Could you check a few things on this model? Use its own coordinates, in mm. Face numbers are marked on the shaded views. A direction names the side the tool comes from. Coordinates: 2 decimals unless noted, no trailing zeros. Loops run counter-clockwise (first coordinate to the right, second up) from the corner with the lowest first, then second, coordinate; pieces in that order, holes last. Notation, with made-up numbers: M 86,40.25 L 141,40.25 A20 cw 141,73.25 Z; hole C 88,23 d6. An arc over 180 degrees is marked long. Write each question's results on one line, items separated by ' | '.
```python
from build123d import *

# Parameters (mm, degrees)
SKETCH1_R           = 10.16
BOSS_EXTRUDE1_DEPTH = 7.62
SKETCH2_R           = 1.5875
CUT_EXTRUDE4_DEPTH  = 17.263935563
CUT_EXTRUDE5_DEPTH  = 6.35


with BuildPart() as part:
    # Sketch1 → Boss-Extrude1 (new body)
    with BuildSketch(Plane(origin=(0, 0, 0), x_dir=(1, 0, 0), z_dir=(0, 1, 0))):
        with Locations(Location((0, 0, 0), (0, 0, 90))):
            Circle(SKETCH1_R)
    extrude(amount=BOSS_EXTRUDE1_DEPTH)

    # Sketch2 → Cut-Extrude4 (cut, through all)
    with BuildSketch(Plane(origin=(0, 7.62, 0), x_dir=(1, 0, 0), z_dir=(0, 1, 0))):
        with Locations(Location((0, 0, 0), (0, 0, 270))):
            Circle(SKETCH2_R)
    extrude(amount=-CUT_EXTRUDE4_DEPTH, mode=Mode.SUBTRACT)

    # Sketch5 → Cut-Extrude5 (cut)
    with BuildSketch(Plane(origin=(0, 7.62, 0), x_dir=(1, 0, 0), z_dir=(0, 1, 0))):
        Polygon((6.247359776, 1.137099745), (2.138922622, 5.978922145), (-4.108437154, 4.8418224), (-6.247359776, -1.137099745), (-2.138922622, -5.978922145), (4.108437154, -4.8418224), align=None)
    extrude(amount=-CUT_EXTRUDE5_DEPTH, mode=Mode.SUBTRACT)


solid = part.part
```
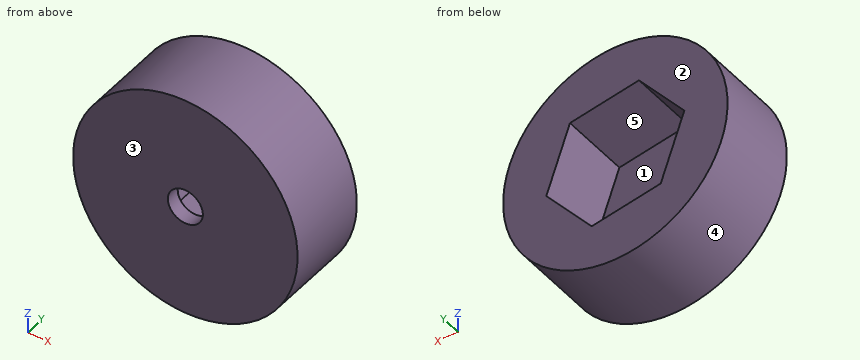
(1) Imagine slicing it at B-B, the plane y = 2.5. List the corners of the cut face in (x, z) for me, and give its area (3 significant figures).
Reported:
outline: C 0,0 d20.32; hole M -6.25,1.14 L -4.11,-4.84 L 2.14,-5.98 L 6.25,-1.14 L 4.11,4.84 L -2.14,5.98 Z | area: 220 mm2
(2) Imagine slicing it at C-C, the plane x = -5. List the corners of the cut face in (y, z) for me.
Reported:
outline: M 0,-8.84 L 7.62,-8.84 L 7.62,-2.35 L 1.27,-2.35 L 1.27,2.61 L 7.62,2.61 L 7.62,8.84 L 0,8.84 Z
(3) If we mould it in two halves opening along X, with no side actions, what happens to the marked faces 3, 4 and 5? For each: released by +X, released by -X, zero draft, split by the parting line, or undercut.
Reported:
face 3: zero draft | face 4: split by the parting line | face 5: undercut
(4) Please list where these lines run through material, in increasing order: probe 1 along X at (y, z) = (0.5, 0); probe 2 along X at (y, z) = (5.25, 0.25); probe 3 along Z at (x, y) = (1.25, 6.5). Write a range as from..to.
Reported:
probe 1: x = -10.16..-1.59, 1.59..10.16 | probe 2: x = -10.16..-5.93, 5.75..10.16 | probe 3: z = -10.08..-5.82, 5.36..10.08
(5) Will these pins go through, and if not, where does the flat tip stop? P1, Ø1.5, axis at y = 6.5, z = 2, coming from the +X side; P2, Ø1, axis at x = 3.5, y = 3, coming from the +Z side; P3, Ø3, axis at y = 6, z = 5.5, coming from the +X side; P4, Ø2.5, axis at x = 0, z = 0, coming from the -Y side.
Reported:
P1: stops at x = 10.08 | P2: stops at z = 9.71 | P3: stops at x = 9.34 | P4: passes through
(6) Which directions (+Z, -Z, +X, -X, +Y, -Y) give clear straight access to the entire face, cutting with the end or side of a thin tool? Please do the marked faces 1 and 2.
Reported:
face 1: +Y | face 2: +Z, -Z, +X, -X, +Y
(7) Imagine slicing it at A-A, the plane z = 0. List the corners of the cut face in (x, y) for me.
Reported:
outline: M -10.16,0 L -1.59,0 L -1.59,1.27 L -5.84,1.27 L -5.84,7.62 L -10.16,7.62 Z; M 1.59,0 L 10.16,0 L 10.16,7.62 L 5.84,7.62 L 5.84,1.27 L 1.59,1.27 Z
(8) Imagine slicing it at D-D, the plane x = 0. List the corners of the cut face in (y, z) for me.
Reported:
outline: M 0,-10.16 L 7.62,-10.16 L 7.62,-5.59 L 1.27,-5.59 L 1.27,-1.59 L 0,-1.59 Z; M 0,1.59 L 1.27,1.59 L 1.27,5.59 L 7.62,5.59 L 7.62,10.16 L 0,10.16 Z
